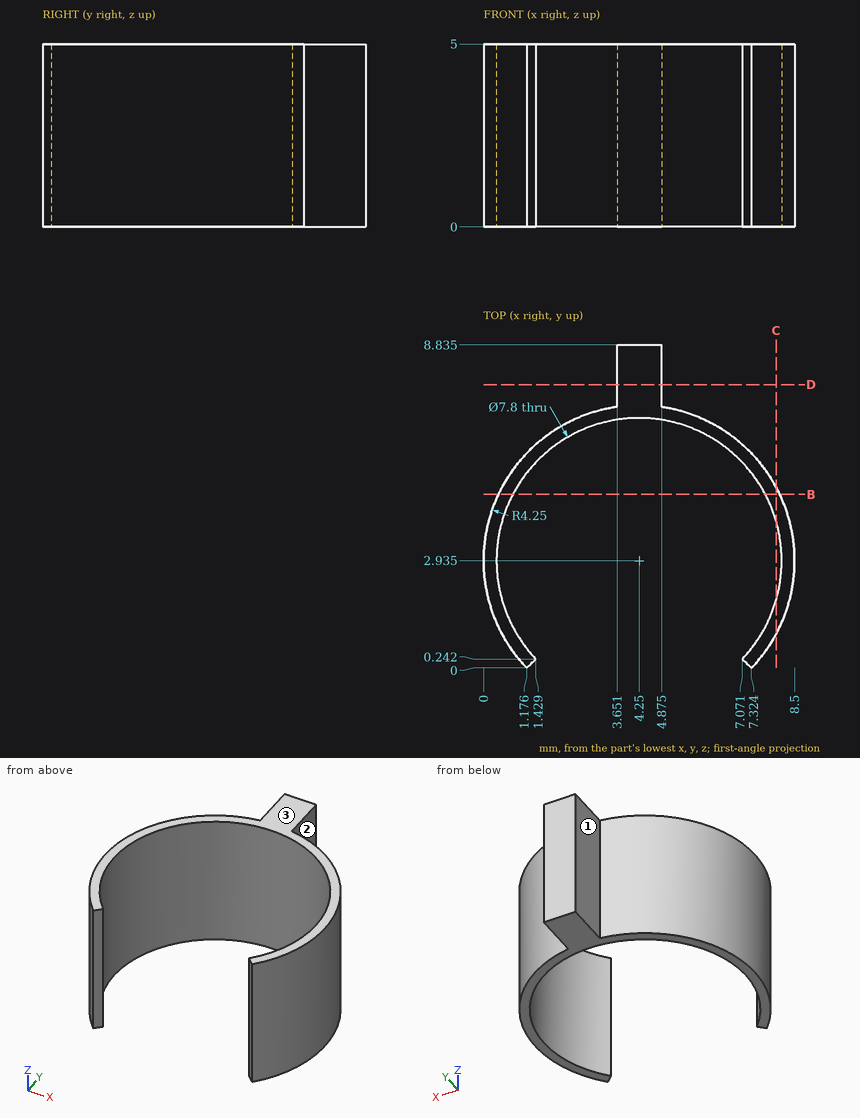
Study the drawing (mm; zero at the part's minimum x, y, z) and answer. A direction names the side the tool comes from. Coordinates: 2 decimals unless noted, no trailing zeros. Write each loop counter-clockwise with the first axis right and the second up, starting at its lowest first coordinate (ties: lowest second). Pieces come first, ordered by that corner, then holes. Notation, with made-up numbers: (76, 39) - (88, 39) arc R20 cw to (88, 64) - close; hole circle Ø1 at (61.25, -29). An arc over 180 degrees is marked (long way). One line per item, written item: value.
1) Each of these flat-tipped pins is pushed along its axis until it touches: pin 1 Ø2 at (x, z) = (5, 2) entering from -Y; pin 2 Ø3 at (x, y) = (5, 7.5) entering from -Z; pin 3 Ø4.5 at (x, y) = (4.25, 2.93) entering from +Z; pin 4 Ø0.8 at (y, z) = (8, 2) entering from +X (3 decimals). Where does it stop, or does it pass through?
Geometry check:
pin 1: stops at y = 6.42
pin 2: stops at z = 0
pin 3: passes through
pin 4: stops at x = 4.875
2) Consider line 1 along X through (y, z) = (3, 2.75); line 2 along X through (y, z) = (8.75, 4.5) (1 decimal); line 3 along X through (y, z) = (3.75, 1.3). Determine where each line is inside the solid, lowest interval first. Write a range as from..to.
Geometry check:
line 1: x = 0..0.35, 8.15..8.5
line 2: x = 3.7..4.9
line 3: x = 0.08..0.44, 8.06..8.42
3) Find section B-B (y = 4.75). Give the vertices of the cut face in (x, z).
Geometry check:
outline: (0.41, 0) - (0.8, 0) - (0.8, 5) - (0.41, 5) - close; (7.7, 0) - (8.09, 0) - (8.09, 5) - (7.7, 5) - close
4) Find section C-C (x = 8). Give the vertices of the cut face in (y, z) (1 decimal).
Geometry check:
outline: (0.9, 0) - (1.9, 0) - (1.9, 5) - (0.9, 5) - close; (4, 0) - (4.9, 0) - (4.9, 5) - (4, 5) - close
5) Find section D-D (y = 7.75). Give the vertices of the cut face in (x, z) (1 decimal).
Geometry check:
outline: (3.7, 0) - (4.9, 0) - (4.9, 5) - (3.7, 5) - close
6) A tool of negligible diameter and unlimited length cuts with its end or side. For the marked faces 1, 2 and 3, from which of +Z, -Z, +X, -X, +Y, -Y can it reach the whole face along a straight path? Write none if from no direction.
Geometry check:
face 1: +Z, -Z, -X, +Y
face 2: +Z, -Z, +X, +Y
face 3: +Z, +X, -X, +Y, -Y
